For this review, take the finished solid that the model builds, in its own axes (mm). A direction names the side the tool comes from. Coordinates: 2 decimals unless noted, no trailing zeros. Write each loop counter-clockwise with the first axis right and the second up, starting at its lowest first coordinate (ties: lowest second). Pieces come first, ordered by that corner, then holes. Notation, with made-up numbers: (57, 9) - (114, 9) arc R19 cw to (114, 39) - close; hole circle Ø2 at (-3, -25). An arc over 180 degrees is marked (long way). Write each question's results on one line, items separated by ' | '.
from build123d import *

# Parameters (mm, degrees)
BOSS_EXTRUDE4_DEPTH      = 40
BOSS_EXTRUDE4_DEPTH_BACK = 20
SKETCH5_OUTSIDE_W        = 102.574
SKETCH5_OUTSIDE_H        = 142.574
CUT_EXTRUDE1_DEPTH       = 348.961204734
SKETCH6_R                = 1.6
CUT_EXTRUDE2_DEPTH       = 346.049136601
FILLET1_R                = 4
SKETCH7_R                = 3.2
CUT_EXTRUDE3_DEPTH       = 3


with BuildPart() as part:
    # Sketch4 → Boss-Extrude4 (new, two sides: drawn at the far end of the back side and taken through both)
    with BuildSketch(Plane(origin=(0, 0, -249), x_dir=(-1, 0, 0), z_dir=(0, 0, -1)).offset(-BOSS_EXTRUDE4_DEPTH_BACK)):
        with BuildLine():
            Line((-83, 0), (-83, 34.267002189))
            ThreePointArc((-83, 34.267002189), (-82.659258263, 36.85519264), (-81.660254038, 39.267002189))
            Line((-81.660254038, 39.267002189), (-53.812919768, 87.5))
            ThreePointArc((-53.812919768, 87.5), (-44.662284673, 96.650635095), (-32.162284673, 100))
            Line((-32.162284673, 100), (0, 100))
            Line((0, 100), (32.162284673, 100))
            ThreePointArc((32.162284673, 100), (44.662284673, 96.650635095), (53.812919768, 87.5))
            Line((53.812919768, 87.5), (81.660254038, 39.267002189))
            ThreePointArc((81.660254038, 39.267002189), (82.659258263, 36.85519264), (83, 34.267002189))
            Line((83, 34.267002189), (83, 0))
            Line((83, 0), (80, 0))
            Line((80, 0), (80, 34.267002189))
            ThreePointArc((80, 34.267002189), (79.761480784, 36.078735505), (79.062177826, 37.767002189))
            Line((79.062177826, 37.767002189), (51.214843556, 86))
            ThreePointArc((51.214843556, 86), (43.162284673, 94.052558883), (32.162284673, 97))
            Line((32.162284673, 97), (0, 97))
            Line((0, 97), (-32.162284673, 97))
            ThreePointArc((-32.162284673, 97), (-43.162284673, 94.052558883), (-51.214843556, 86))
            Line((-51.214843556, 86), (-79.062177826, 37.767002189))
            ThreePointArc((-79.062177826, 37.767002189), (-79.761480784, 36.078735505), (-80, 34.267002189))
            Line((-80, 34.267002189), (-80, 0))
            Line((-80, 0), (-83, 0))
        make_face()
    extrude(amount=BOSS_EXTRUDE4_DEPTH + BOSS_EXTRUDE4_DEPTH_BACK)

    # Sketch5 outside → Cut-Extrude1 (cut, through all)
    with BuildSketch(Plane(origin=(83, 0, 0), x_dir=(0, 0, -1), z_dir=(1, 0, 0))):
        with Locations((259, 50)):
            Rectangle(SKETCH5_OUTSIDE_W, SKETCH5_OUTSIDE_H)
        with BuildLine():
            Line((229, 100), (254.037739827, 37.863968909))
            ThreePointArc((254.037739827, 37.863968909), (255.121445979, 34.196094194), (255.487139078, 30.388996545))
            Line((255.487139078, 30.388996545), (255.487139078, 0))
            Line((255.487139078, 0), (285.487139078, 0))
            Line((285.487139078, 0), (285.487139078, 30.388996545))
            ThreePointArc((285.487139078, 30.388996545), (285.121445979, 34.196094194), (284.037739827, 37.863968909))
            Line((284.037739827, 37.863968909), (259, 100))
            Line((259, 100), (229, 100))
        make_face(mode=Mode.SUBTRACT)
    extrude(amount=-CUT_EXTRUDE1_DEPTH, mode=Mode.SUBTRACT)

    # Sketch6 → Cut-Extrude2 (cut, through all)
    with BuildSketch(Plane(origin=(83, 0, 0), x_dir=(0, 0, -1), z_dir=(1, 0, 0))):
        with Locations((262.487139078, 8)):
            Circle(SKETCH6_R)
        with Locations((278.487139078, 8)):
            Circle(SKETCH6_R)
    extrude(amount=-CUT_EXTRUDE2_DEPTH, mode=Mode.SUBTRACT)

    # Fillet1
    fillet1_edges = [part.edges().sort_by_distance(p)[0] for p in [
        (81.5, 0, -285.487139078),
        (-81.5, 0, -285.487139078),
        (81.5, 0, -255.487139078),
        (-81.5, 0, -255.487139078),
    ]]
    fillet(fillet1_edges, radius=FILLET1_R)

    # Sketch7 → Cut-Extrude3 (cut)
    with BuildSketch(Plane(origin=(0, 100, 0), x_dir=(1, 0, 0), z_dir=(0, 1, 0))):
        with Locations(Location((-20.162284673, 244, 0), (0, 0, 270))):
            Circle(SKETCH7_R)
        with Locations(Location((20.162284673, 244, 0), (0, 0, 270))):
            Circle(SKETCH7_R)
    extrude(amount=-CUT_EXTRUDE3_DEPTH, mode=Mode.SUBTRACT)


solid = part.part
Q1. Mouldability with a two-part tool opening along Z and no side actions: class faces 1 (the face through (43.022, 94.133, -247.184)), 2 (the face through (-81.521, 1.203, -284.346)), 3 (the face through (81.47, 34.25, -255.11)), 4 (the face through (21.123, 98.521, -240.948)) as pulls with the +Z half, pulls with the -Z half, needs draft (parallel to the pull), parting line crosses it, or undercut.
Results found:
face 1: needs draft | face 2: pulls with the -Z half | face 3: pulls with the +Z half | face 4: undercut
Q2. Wall thickness on line 1 along X through (y, z) = (5.5, -274); line 2 along Y through (x, z) = (22.5, -254.5); line 3 along X through (y, z) = (74, -250.5): over which ranges is each line inside the solid? List them lowest first. Write a range as from..to.
Results found:
line 1: -83..-80, 80..83 | line 2: 97..100 | line 3: -61.61..-58.14, 58.14..61.61
Q3. Take a section at A-A on y = 28. State the section outline as (x, z) points.
Results found:
outline: (-83, -285.49) - (-80, -285.49) - (-80, -255.49) - (-83, -255.49) - close; (80, -285.49) - (83, -285.49) - (83, -255.49) - (80, -255.49) - close
Q4. Take a section at D-D on x = 57. State the section outline as (y, z) points, plus the area to 3 significant figures.
Results found:
outline: (75.98, -268.68) - (81.98, -266.26) - (81.98, -236.26) - (75.98, -238.68) - close | area: 180 mm2
Q5. Take a section at B-B on z = -244. State the section outline as (x, y) points, plus the area to 3 significant figures.
Results found:
outline: (-68.09, 62.77) - (-64.62, 62.77) - (-51.21, 86) arc R22 cw to (-32.16, 97) - (-23.36, 97) - (-23.36, 100) - (-32.16, 100) arc R25 ccw to (-53.81, 87.5) - close; (-16.96, 97) - (16.96, 97) - (16.96, 100) - (-16.96, 100) - close; (23.36, 97) - (32.16, 97) arc R22 cw to (51.21, 86) - (64.62, 62.77) - (68.09, 62.77) - (53.81, 87.5) arc R25 ccw to (32.16, 100) - (23.36, 100) - close | area: 468 mm2
Q6. For faces 5 (the face through (0.384, 98.994, -229.405)), 6 (the face through (79.755, 36.104, -269.375)), list the 3-axis set-ups (+Z, -Z, +X, -X, +Y, -Y) from which the entire face can be reached by the end or side of a thin tool; tool diameter is ignored.
Results found:
face 5: +Z, +X, -X, -Y | face 6: +Z, -Z, -Y
Q7. For pin 1 (1 mm diameter, centred on y = 84, z = -248, fed in from +X); pin 2 (24 mm diameter, centred on x = 5, z = -247, fed in from -Y); pin 3 (1.5 mm diameter, centred on x = -82, y = 21.5, fed in from +Z); pin 4 (3 mm diameter, centred on y = 8, z = -262.49, fed in from -X), all flat-tipped, find the tip position at first contact; note any pin that passes through.
Results found:
pin 1: x = 56.12 | pin 2: y = 97 | pin 3: z = -255.49 | pin 4: through
Q8. Take a section at C-C on y = 53.5. State the section outline as (x, z) points, plus the area to 3 significant figures.
Results found:
outline: (-73.44, -277.74) - (-69.98, -277.74) - (-69.98, -247.74) - (-73.44, -247.74) - close; (69.98, -277.74) - (73.44, -277.74) - (73.44, -247.74) - (69.98, -247.74) - close | area: 208 mm2
